Input: part model. Units: mm. Frame: model coordinates. A direction names the side the tool comes from. Give positions to 0.01 mm unless a question says otherwise; leave off trailing zeros. Order: outer loops, then holes, each group sorted by start corner. A loop starts at its lowest first (then second) coordinate and runs counter-clockwise, first axis right, second up. Notation, with made-up numbers: (37, 43) - (95, 43) arc R19 ccw to (95, 78) - close; hole circle Ø5 at (9, 28). An arc over 180 degrees is marked (long way). Answer in a Markdown table with one row per item. Add a question column.
1. Mould query, pull axis Z, two halves, no side actions, for faces 1 (the face through (-448.46, -227.32, 2.46)), 2 (the face through (-460, -186.231, 67)), 3 (the face through (-447, -202, 89)). Classes: released by +Z, released by -Z, zero draft, split by the parting line, or undercut.
2. Section query C-C on z = 72. Return loops of the section in (x, y).
3. Ray query, line 1 (X direction, y = -185.5, z = 34.5); line 2 (Z direction, x = -450, y = -213.5); line 3 (Y direction, x = -460, z = 14). Return the intervals inside material, ascending. Write a range as [from, to].
4. Access query for faces 4 (the face through (-461, -224.081, 24)), 5 (the face through (-461, -181.581, 24)), 6 (the face through (-437, -203, 5)), 7 (the face through (-442, -193.863, 67)). Directions: +Z, -Z, +X, -X, +Y, -Y. A direction counts if a zero-diameter tool reaches every point of the face in a straight line with its end or side. Return the directions, or none.
5. Contact query for flat-ended pins moving along their axis: pin 1 (12 mm diameter, centred on x = -442.5, z = 13.5, fed in from -Y); pin 2 (2 mm diameter, centred on x = -455.5, z = 48, fed in from +Y); pin 3 (5.5 mm diameter, centred on x = -456, z = 60.5, fed in from +Y). Output: stop coordinate, or through.
6. Section query D-D on z = 21. Return loops of the section in (x, y), and give its area (4 significant figures).
```python
from build123d import *

# Parameters (mm, degrees)
SKETCH6_R           = 1.5
BOSS_EXTRUDE4_DEPTH = 5
SKETCH8_W           = 44.5
SKETCH8_H           = 44.5
SKETCH8_R           = 1.5
SKETCH8_R_2         = 12.5
BOSS_EXTRUDE5_DEPTH = 50
SKETCH7_W           = 43.5
SKETCH7_H           = 42.5
CUT_EXTRUDE4_DEPTH  = 48.25
BOSS_EXTRUDE6_DEPTH = 1
SKETCH11_W          = 18
SKETCH11_H          = 4.15
SKETCH11_W_2        = 4.15
SKETCH11_H_2        = 18
BOSS_EXTRUDE7_DEPTH = 35
SKETCH14_W          = 60
SKETCH14_H          = 60
BOSS_EXTRUDE8_DEPTH = 4
CUT_EXTRUDE5_REACH  = 551.669
SKETCH16_R          = 2.5
SKETCH17_R          = 12.5
CUT_EXTRUDE6_DEPTH  = 550.668785806


with BuildPart() as part:
    # Sketch6 → Boss-Extrude4 (new body)
    with BuildSketch(Plane.XY):
        Polygon((-437.521213625, -225.081134847), (-482.021213625, -225.081134847), (-482.021213625, -232.581134847), (-430.021213625, -232.581134847), (-430.021213625, -173.081134847), (-482.021213625, -173.081134847), (-482.021213625, -180.581134847), (-437.521213625, -180.581134847), align=None)
        with Locations((-464.687880625, -228.331134847)):
            Circle(SKETCH6_R, mode=Mode.SUBTRACT)
        with Locations((-447.354547625, -228.331134847)):
            Circle(SKETCH6_R, mode=Mode.SUBTRACT)
        with Locations((-434.271213625, -211.715651861)):
            Circle(SKETCH6_R, mode=Mode.SUBTRACT)
        with Locations((-464.687883625, -176.831134847)):
            Circle(SKETCH6_R, mode=Mode.SUBTRACT)
        with Locations((-434.271213625, -194.382318861)):
            Circle(SKETCH6_R, mode=Mode.SUBTRACT)
        with Locations((-447.354550625, -176.831134847)):
            Circle(SKETCH6_R, mode=Mode.SUBTRACT)
    extrude(amount=BOSS_EXTRUDE4_DEPTH)

    # Sketch8 → Boss-Extrude5 (add)
    with BuildSketch(Plane.XY):
        with Locations((-459.771213625, -202.831134847)):
            Rectangle(SKETCH8_W, SKETCH8_H)
        with Locations((-475.271213625, -218.331134847)):
            Circle(SKETCH8_R, mode=Mode.SUBTRACT)
        with Locations((-444.271213625, -218.331134847)):
            Circle(SKETCH8_R, mode=Mode.SUBTRACT)
        with Locations((-444.271213625, -187.331134847)):
            Circle(SKETCH8_R, mode=Mode.SUBTRACT)
        with Locations((-475.271213625, -187.331134847)):
            Circle(SKETCH8_R, mode=Mode.SUBTRACT)
        with Locations((-460.021213625, -202.581134847)):
            Circle(SKETCH8_R_2, mode=Mode.SUBTRACT)
    extrude(amount=BOSS_EXTRUDE5_DEPTH)

    # Sketch7 → Cut-Extrude4 (cut)
    with BuildSketch(Plane.XY):
        with Locations((-460.271213625, -202.831134847)):
            Rectangle(SKETCH7_W, SKETCH7_H)
    extrude(amount=CUT_EXTRUDE4_DEPTH, mode=Mode.SUBTRACT)

    # Sketch10 → Boss-Extrude6 (add)
    with BuildSketch(Plane.ZY.offset(482.021213625)):
        Polygon((24.125, -181.581134847), (48.25, -224.081134847), (48.25, -181.581134847), align=None)
    extrude(amount=-BOSS_EXTRUDE6_DEPTH)

    # Sketch11 → Boss-Extrude7 (add)
    with BuildSketch(Plane.XY.offset(50)):
        with Locations((-460.303059696, -221.006134847)):
            Rectangle(SKETCH11_W, SKETCH11_H)
        with Locations((-441.596213625, -202.862980918)):
            Rectangle(SKETCH11_W_2, SKETCH11_H_2)
        with Locations((-478.446213625, -202.299288776)):
            Rectangle(SKETCH11_W_2, SKETCH11_H_2)
        with Locations((-459.739367554, -184.156134847)):
            Rectangle(SKETCH11_W, SKETCH11_H)
    extrude(amount=BOSS_EXTRUDE7_DEPTH)

    # Sketch14 → Boss-Extrude8 (add)
    with BuildSketch(Plane.XY.offset(85)):
        with Locations((-460.021213625, -202.581134847)):
            Rectangle(SKETCH14_W, SKETCH14_H)
    extrude(amount=BOSS_EXTRUDE8_DEPTH)

    # Sketch16 → Cut-Extrude5 (cut, up to next)
    with BuildSketch(Plane.XY.offset(89), mode=Mode.PRIVATE) as cut_extrude5_sk1:
        with Locations((-447.116514868, -189.67643609)):
            Circle(SKETCH16_R)
    cut_extrude5_tool1 = extrude(cut_extrude5_sk1.sketch, amount=-CUT_EXTRUDE5_REACH, mode=Mode.PRIVATE) & part.part
    # Sketch16 → Cut-Extrude5 (cut, up to next)
    with BuildSketch(Plane.XY.offset(89), mode=Mode.PRIVATE) as cut_extrude5_sk2:
        with Locations((-472.925912382, -215.485833604)):
            Circle(SKETCH16_R)
    cut_extrude5_tool2 = extrude(cut_extrude5_sk2.sketch, amount=-CUT_EXTRUDE5_REACH, mode=Mode.PRIVATE) & part.part
    add(cut_extrude5_tool1.solids().sort_by_distance((-447.116515, -189.676436, 89))[0], mode=Mode.SUBTRACT)
    add(cut_extrude5_tool2.solids().sort_by_distance((-472.925912, -215.485834, 89))[0], mode=Mode.SUBTRACT)

    # Sketch17 → Cut-Extrude6 (cut, through all)
    with BuildSketch(Plane.XY):
        with Locations(Location((-460.021213625, -202.581134847, 0), (0, 0, 180))):
            Circle(SKETCH17_R)
    extrude(amount=CUT_EXTRUDE6_DEPTH, mode=Mode.SUBTRACT)


solid = part.part
```
Answer:
| question | item | result |
|---|---|---|
| 1 | face 1 | zero draft |
| 1 | face 2 | undercut |
| 1 | face 3 | released by +Z |
| 2 | outline | (-480.52, -211.3) - (-476.37, -211.3) - (-476.37, -193.3) - (-480.52, -193.3) - close; (-469.3, -223.08) - (-451.3, -223.08) - (-451.3, -218.93) - (-469.3, -218.93) - close; (-468.74, -186.23) - (-450.74, -186.23) - (-450.74, -182.08) - (-468.74, -182.08) - close; (-443.67, -211.86) - (-439.52, -211.86) - (-439.52, -193.86) - (-443.67, -193.86) - close |
| 3 | line 1 | x = [-482.02, -481.02], [-438.52, -437.52] |
| 3 | line 2 | z = [48.25, 50], [85, 89] |
| 3 | line 3 | y = [-225.08, -224.08], [-181.58, -180.58] |
| 4 | face 4 | -Z, -X |
| 4 | face 5 | -Z |
| 4 | face 6 | +X |
| 4 | face 7 | +X, +Y |
| 5 | pin 1 | stops at y = -225.08 |
| 5 | pin 2 | stops at y = -180.58 |
| 5 | pin 3 | stops at y = -182.08 |
| 6 | outline | (-482.02, -225.08) - (-437.52, -225.08) - (-437.52, -180.58) - (-482.02, -180.58) - (-482.02, -181.58) - (-438.52, -181.58) - (-438.52, -224.08) - (-482.02, -224.08) - close |
| 6 | area | 131.5 mm² |
